Read the model definition and answer for the solid it produces. Units are mm, in the model's axes. Face numbers are marked on the shaded views. A direction names the side the tool comes from. Coordinates: 2 decimals unless noted, no trailing zeros. Loops run counter-clockwise (first coordinate to the right, second up) from the corner with the lowest first, then second, coordinate; pieces in that order, holes last. Notation, with made-up numbers: (-28.75, -17) -> (20.25, -17) arc R24 ccw to (20.25, 16) -> close; hole circle Ø3 at (34.5, 62). An arc over 180 degrees is marked (long way). Answer as a JSON object with one key per item and string values. Group by question number.
1) Section C-C, the plane x = 0.5 is taken. Give the vertices of the cut face in (y, z), plus the area to 3 significant figures.
2) Flat-ended cylindrical pins translate along their axes: P1, Ø1, axis at x = -0.5, y = -4.5, coming from the +Z side; P2, Ø1.5, axis at x = 0, z = -1.5, coming from the +Y side; P3, Ø2, axis at x = -1.5, z = 3.5, coming from the +Y side. Find the tip coordinate at first contact, or state that the pin passes through.
3) Section D-D, the plane x = -2 is taken. Give the vertices of the cut face in (y, z).
4) Section B-B, the plane y = -1.2 is taken. Give the vertices of the cut face in (x, z), plus the area to 3 significant figures.
5) Which of the six approach directions +Z, -Z, +X, -X, +Y, -Y give full straight-line access (tool end or side, diameter ignored) to the marked faces 1, 2 and 3?
6) Section A-A, the plane z = -0.5 is taken. Give the vertices of the cut face in (x, y).
7) Consider probe 1 along X at (y, z) = (-3, 3.5); probe 2 along Y at (x, z) = (-1.2, 0.25); probe 3 along Y at (x, z) = (-0.3, -0.5). Determine where each line is inside the solid, lowest interval first. Write a range as [from, to].
8) Determine the mould class of the marked faces 4, 5, 6 and 7 for opening direction X: released by +X, released by -X, zero draft, split by the parting line, or undercut.
from build123d import *

# Parameters (mm, degrees)
FILLET_1_R = 1.2


with BuildPart() as part:
    # По траектории2: sweep along a path in Эскиз3
    with BuildLine(Plane(origin=(0, 0, 0), x_dir=(0, 0, -1), z_dir=(1, 0, 0))) as sweep_2_path:
        Line((-1, 0), (1, 0))
        ThreePointArc((1, 0), (2.2, -1.2), (1, -2.4))
        Line((1, -2.4), (-1, -2.4))
        ThreePointArc((-1, -2.4), (-2.2, -1.2), (-1, 0))
    # Эскиз1 → По траектории2 (sweep)
    with BuildSketch(Plane.XY):
        Polygon((-0.8, 1), (0.8, 1), (0.8, 3.25), (2.5, 3.25), (2.5, 0), (-2.5, 0), (-2.5, 3.25), (-0.8, 3.25), align=None)
    sweep(path=sweep_2_path.line)

    # Скругление1
    fillet_1_edges = [part.edges().sort_by_distance(p)[0] for p in [
        (2.5, 3.25, 0),
        (-2.5, 3.25, 0),
        (2.5, -1.2, 5.45),
        (-2.5, -1.2, 5.45),
        (2.5, -5.65, 0),
        (-2.5, -5.65, 0),
        (2.5, -1.2, -5.45),
        (-2.5, -1.2, -5.45),
    ]]
    fillet(fillet_1_edges, radius=FILLET_1_R)


solid = part.part
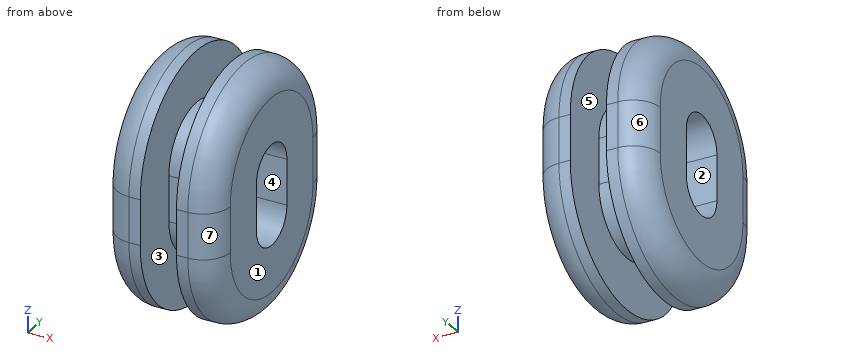
Determined:
{
 "1": {"outline": "(-3.4, -1) arc R2.2 ccw to (1, -1) -> (1, 1) arc R2.2 ccw to (-3.4, 1) -> close; hole (-2.4, -1) arc R1.2 ccw to (0, -1) -> (0, 1) arc R1.2 ccw to (-2.4, 1) -> close", "area": "14.7 mm²"},
 "2": {"P1": "z = 4.38", "P2": "y = 1", "P3": "y = 2.98"},
 "3": {"outline": "(-5.42, -1) arc R4.22 ccw to (3.02, -1) -> (3.02, 1) arc R4.22 ccw to (-5.42, 1) -> close; hole (-2.4, -1) arc R1.2 ccw to (0, -1) -> (0, 1) arc R1.2 ccw to (-2.4, 1) -> close"},
 "4": {"outline": "(-2.5, -4.25) arc R1.2 ccw to (-1.3, -5.45) -> (-0.8, -5.45) -> (-0.8, -3.2) -> (0.8, -3.2) -> (0.8, -5.45) -> (1.3, -5.45) arc R1.2 ccw to (2.5, -4.25) -> (2.5, -2.2) -> (-2.5, -2.2) -> close; (-2.5, 2.2) -> (2.5, 2.2) -> (2.5, 4.25) arc R1.2 ccw to (1.3, 5.45) -> (0.8, 5.45) -> (0.8, 3.2) -> (-0.8, 3.2) -> (-0.8, 5.45) -> (-1.3, 5.45) arc R1.2 ccw to (-2.5, 4.25) -> close", "area": "24.1 mm²"},
 "5": {"face 1": "+Z, -Z, +X, +Y, -Y", "face 2": "+X, -X", "face 3": "none"},
 "6": {"outline": "(-2.5, -4.45) arc R1.2 ccw to (-1.3, -5.65) -> (-0.8, -5.65) -> (-0.8, -3.4) -> (0.8, -3.4) -> (0.8, -5.65) -> (1.3, -5.65) arc R1.2 ccw to (2.5, -4.45) -> (2.5, -2.4) -> (-2.5, -2.4) -> close; (-2.5, 0) -> (2.5, 0) -> (2.5, 2.05) arc R1.2 ccw to (1.3, 3.25) -> (0.8, 3.25) -> (0.8, 1) -> (-0.8, 1) -> (-0.8, 3.25) -> (-1.3, 3.25) arc R1.2 ccw to (-2.5, 2.05) -> close"},
 "7": {"probe 1": "[-2.5, -0.8], [0.8, 2.5]", "probe 2": "[-5.65, -2.4], [0, 3.25]", "probe 3": "[-3.4, -2.4], [0, 1]"},
 "8": {"face 4": "zero draft", "face 5": "undercut", "face 6": "released by -X", "face 7": "released by +X"}
}
